from build123d import *

# Parameters (mm, degrees)
SKETCH1_W           = 22.5
SKETCH1_H           = 38
BOSS_EXTRUDE1_DEPTH = 2
SKETCH2_W           = 7
SKETCH2_H           = 22
BOSS_EXTRUDE2_DEPTH = 4
SKETCH3_R           = 2.706246926
SKETCH3_W           = 7.563295119
SKETCH3_H           = 10.529749536
BOSS_EXTRUDE3_DEPTH = 2
SKETCH4_W           = 3.522294841
SKETCH4_H           = 18.892308692
CUT_EXTRUDE1_DEPTH  = 6
SKETCH5_R           = 5
BOSS_EXTRUDE4_DEPTH = 20
SKETCH6_OUTSIDE_W   = 37.102
SKETCH6_OUTSIDE_H   = 24.602
SKETCH6_OUTSIDE_W_2 = 2.5
SKETCH6_OUTSIDE_H_2 = 9.5
CUT_EXTRUDE2_DEPTH  = 12
SKETCH7_R           = 5
BOSS_EXTRUDE5_DEPTH = 80
BOSS_EXTRUDE5_DRAFT = -1


with BuildPart() as part:
    # Sketch1 → Boss-Extrude1 (new body)
    with BuildSketch(Plane.XY):
        Rectangle(SKETCH1_W, SKETCH1_H)
    extrude(amount=BOSS_EXTRUDE1_DEPTH)

    # Sketch2 → Boss-Extrude2 (add)
    with BuildSketch(Plane.XY.offset(2)):
        with Locations((-7.75, -6.011083038)):
            Rectangle(SKETCH2_W, SKETCH2_H)
    extrude(amount=BOSS_EXTRUDE2_DEPTH)

    # Sketch3 → Boss-Extrude3 (add)
    with BuildSketch(Plane.XY.offset(2)):
        with Locations(Location((-8.15823298, 14.663341742, 0), (0, 0, 180))):
            Circle(SKETCH3_R)
        with Locations((4.035174314, -4.778762907)):
            Rectangle(SKETCH3_W, SKETCH3_H)
    extrude(amount=BOSS_EXTRUDE3_DEPTH)

    # Sketch4 → Cut-Extrude1 (cut)
    with BuildSketch(Plane.ZY.offset(11.25)):
        with Locations((3.240156467, -5.963885583)):
            Rectangle(SKETCH4_W, SKETCH4_H)
    extrude(amount=-CUT_EXTRUDE1_DEPTH, mode=Mode.SUBTRACT)

    # Sketch5 → Boss-Extrude4 (add)
    with BuildSketch(Plane(origin=(0, 19, 0), x_dir=(1, 0, 0), z_dir=(0, 1, 0))):
        with Locations(Location((6.05, -1, 0), (0, 0, 168.463040967))):
            Circle(SKETCH5_R)
    extrude(amount=BOSS_EXTRUDE4_DEPTH)

    # Sketch6 outside → Cut-Extrude2 (cut)
    with BuildSketch(Plane(origin=(0, 39, 0), x_dir=(1, 0, 0), z_dir=(0, 1, 0))):
        with Locations((0, -1)):
            Rectangle(SKETCH6_OUTSIDE_W, SKETCH6_OUTSIDE_H)
        with Locations((6.05, -1)):
            Rectangle(SKETCH6_OUTSIDE_W_2, SKETCH6_OUTSIDE_H_2, mode=Mode.SUBTRACT)
    extrude(amount=-CUT_EXTRUDE2_DEPTH, mode=Mode.SUBTRACT)


with BuildPart() as boss_extrude5_tool:
    # Sketch7 → Boss-Extrude5 (with draft: the straight prism first)
    with BuildSketch(Plane(origin=(0, 0, -3.75), x_dir=(-1, 0, 0), z_dir=(0, 0, -1))):
        with Locations((-6.05, 34)):
            Circle(SKETCH7_R)
    extrude(amount=-BOSS_EXTRUDE5_DEPTH)
    # Boss-Extrude5: the draft: its side faces are tilted about the plane it starts from
    boss_extrude5_sides = [boss_extrude5_tool.faces().sort_by_distance(p)[0] for p in [
        (11.05, 34, 36.25),
    ]]
    draft(boss_extrude5_sides, Plane(origin=(0, 0, -3.75), x_dir=(-1, 0, 0), z_dir=(0, 0, -1)), BOSS_EXTRUDE5_DRAFT)


with BuildPart() as part_1:
    add(part.part)

    # Boss-Extrude5: add boss_extrude5_tool
    add(boss_extrude5_tool.part)


solid = part_1.part
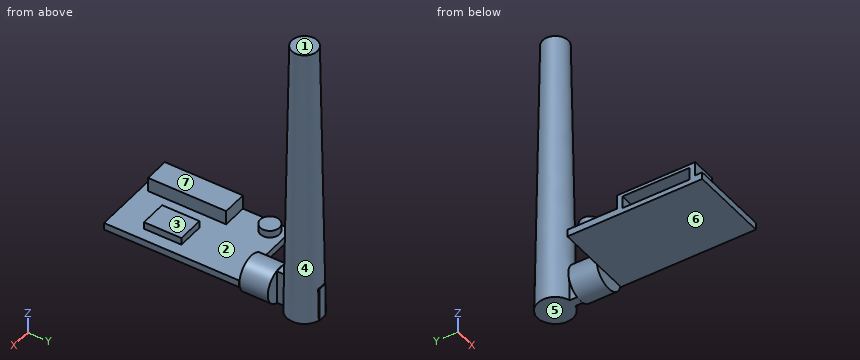
Check sheet for the modelled part. Datum: model origin and axes. Units: mm. Face numbers are marked on the shaded views. A direction names the side the tool comes from. Give positions to 0.01 mm unless a question says otherwise; leave off trailing zeros. Write each loop counter-clockwise with the first axis right and the second up, starting at its lowest first coordinate (ties: lowest second). Pieces come first, ordered by that corner, then holes. Notation, with made-up numbers: (26, -22.5) -> (59, -22.5) arc R19 cw to (59, -12.5) -> close; hole circle Ø9 at (-18, 7.25). An arc over 180 degrees is marked (long way). Use one line per item in the form item = value. Start each with the question number.
1. Thickness scan on line 1 along Z through (x, y) = (-6.75, -3); line 2 along Z through (x, y) = (8, 15.5); line 3 along Y through (x, z) = (5.25, 70.5). Record the ranges inside material, lowest first. Write a range as from..to.
2. Go/stop test with flat-tipped pins: P1, Ø1.6, axis at y = -7, z = 3, coming from the -X side; P2, Ø6.5, axis at x = -8.5, y = -9.5, coming from the -Z side; P3, Ø1.8, axis at x = -9.5, y = -10.5, coming from the +Z side. Record where each tip stops, or that it passes through.
3. Section check D-D (z = 39.5). Record the cut outline in (x, y), and give its area (3 significant figures).
4. Section check A-A (y = -7). Record the cut outline in (x, z).
5. Section check C-C (y = 11). Record the cut outline in (x, z), and give its area (3 significant figures).
6. Access from +Z, -Z, +X, -X, +Y, -Y to the whole of each face (thin tool, end or side, straight path). Record for the marked faces 3, 4, 5, 6 and 7.
7. Mould release check, pull along Y, two halves, no side actions. Record for the marked faces 1 and 2: pulls with the +Y half, pulls with the -Y half, needs draft (parallel to the pull), parting line crosses it, or undercut.
8. Section check B-B (z = 69). Record the cut outline in (x, y).
Conclusion:
q1.line_1 = 0..1.48, 5..6
q1.line_2 = 0..2
q1.line_3 = 30.38..37.62
q2.P1 = -5.25
q2.P2 = 0
q2.P3 = 6
q3.outline = circle Ø8.49 at (6.05, 34)
q3.area = 56.6 mm²
q4.outline = (-11.25, 0) -> (11.25, 0) -> (11.25, 2) -> (7.82, 2) -> (7.82, 4) -> (0.25, 4) -> (0.25, 2) -> (-4.25, 2) -> (-4.25, 6) -> (-11.25, 6) -> (-11.25, 5) -> (-5.25, 5) -> (-5.25, 1.48) -> (-11.25, 1.48) -> close
q5.outline = (-11.25, 0) -> (11.25, 0) -> (11.25, 2) -> (-11.25, 2) -> close
q5.area = 45.0 mm²
q6.face_3 = +Z, +X, -Y
q6.face_4 = +Z
q6.face_5 = -Z, +X, -X, +Y
q6.face_6 = -Z, +X, -X, -Y
q6.face_7 = +Z, +X, -X, +Y, -Y
q7.face_1 = needs draft
q7.face_2 = undercut
q8.outline = circle Ø7.46 at (6.05, 34)
